```python
from build123d import *

# Parameters (mm, degrees)
SKETCH2_W               = 55.351920974
SKETCH2_H               = 25.692475641
SKETCH2_R               = 1.604575537
BOSS_EXTRUDE1_DEPTH     = 2.54
BOSS_EXTRUDE2_START     = 4.355808651
BOSS_EXTRUDE2_OUTLINE_W = 5.429648603
BOSS_EXTRUDE2_OUTLINE_H = 2.54
BOSS_EXTRUDE2_DEPTH     = 8.456135595


# Read off the part's stored shape, not the designer's step: Boss-Extrude2
with BuildPart() as part:
    # Sketch2 → Boss-Extrude1 (new body)
    with BuildSketch(Plane.XY):
        with Locations((27.675960487, 12.846237821)):
            Rectangle(SKETCH2_W, SKETCH2_H)
        with Locations((12.152179379, 2.513985209)):
            Circle(SKETCH2_R, mode=Mode.SUBTRACT)
        with Locations((43.902179379, 2.513985209)):
            Circle(SKETCH2_R, mode=Mode.SUBTRACT)
        with Locations((43.902179379, 22.833985209)):
            Circle(SKETCH2_R, mode=Mode.SUBTRACT)
        with Locations((12.152179379, 22.833985209)):
            Circle(SKETCH2_R, mode=Mode.SUBTRACT)
    extrude(amount=BOSS_EXTRUDE1_DEPTH)

    # Boss-Extrude2 outline → Boss-Extrude2 (add)
    with BuildSketch(Plane.YZ.offset(BOSS_EXTRUDE2_START)):
        with Locations((12.810955728, 3.81)):
            Rectangle(BOSS_EXTRUDE2_OUTLINE_W, BOSS_EXTRUDE2_OUTLINE_H)
    extrude(amount=BOSS_EXTRUDE2_DEPTH)


solid = part.part
```
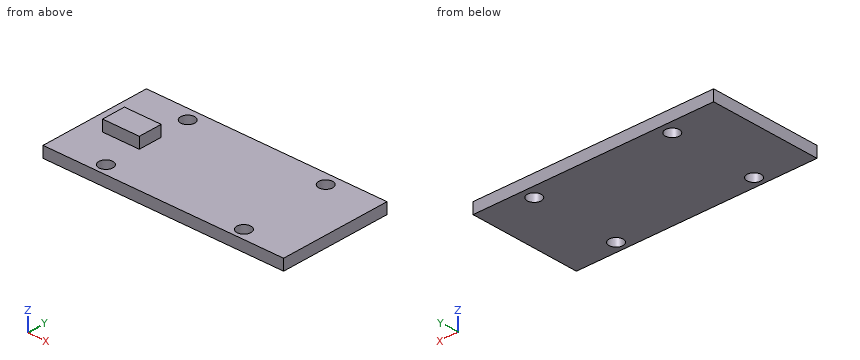
Geometry check sheet. Reference: the model listing, model coordinates, mm. Give positions to 0.01 mm unless a question says otherwise; leave off trailing zeros. Order: outer loops, then holes, each group sorted by start corner. A loop starts at its lowest first (then second) coordinate and runs counter-clockwise, first axis right, second up. Notation, with made-up numbers: (45.5, -2.5) - (90.5, -2.5) arc R20 cw to (90.5, 27.5) - close; hole circle Ø10 at (73.25, 72). An arc over 180 degrees is marked (long way). Write item = value, one per line. Start each with the question number.
1) Section check C-C (z = 1.55). Enter the section's corners in (x, y), then the cut area to 3 significant figures.
2) Gauge pin test, flat ends, axial feed: pin 1 Ø1.9 at (x, y) = (12.15, 22.83) entering from +Z; pin 2 Ø2 at (x, y) = (27.5, 15.5) entering from +Z; pin 3 Ø3.5 at (x, y) = (43.9, 2.51) entering from -Z; pin 4 Ø1.3 at (x, z) = (6.5, 3.5) entering from +Y. Record the tip position at first contact, or that the pin passes through.
3) Section check D-D (x = 26.5). Enter the section's corners in (y, z), then the cut area to 3 significant figures.
4) Section check A-A (y = 14.25). Enter the section's corners in (x, z).
5) Scan lines: L1, parallel to Y at x = 12, z = 1.1; L2, parallel to X at y = 14.25, z = 3.15; L3, parallel to X at y = 24, z = 0.4. Record each from-to range of solid material in increasing order.
6) Section check B-B (x = 44.5). Enter the section's corners in (y, z).
Geometry check:
q1.outline = (0, 0) - (55.35, 0) - (55.35, 25.69) - (0, 25.69) - close; hole circle Ø3.21 at (12.15, 2.51); hole circle Ø3.21 at (12.15, 22.83); hole circle Ø3.21 at (43.9, 2.51); hole circle Ø3.21 at (43.9, 22.83)
q1.area = 1,390 mm2
q2.pin_1 = through
q2.pin_2 = 2.54
q2.pin_3 = 0
q2.pin_4 = 15.53
q3.outline = (0, 0) - (25.69, 0) - (25.69, 2.54) - (0, 2.54) - close
q3.area = 65.3 mm2
q4.outline = (0, 0) - (55.35, 0) - (55.35, 2.54) - (12.81, 2.54) - (12.81, 5.08) - (4.36, 5.08) - (4.36, 2.54) - (0, 2.54) - close
q5.L1 = 0 to 0.92, 4.11 to 21.24, 24.43 to 25.69
q5.L2 = 4.36 to 12.81
q5.L3 = 0 to 11.05, 13.25 to 42.8, 45 to 55.35
q6.outline = (0, 0) - (1.02, 0) - (1.02, 2.54) - (0, 2.54) - close; (4, 0) - (21.34, 0) - (21.34, 2.54) - (4, 2.54) - close; (24.32, 0) - (25.69, 0) - (25.69, 2.54) - (24.32, 2.54) - close
